Autodesk Inventor part; units mm, degrees
ref_plane "YZ Plane" through (0, 0, 0) normal (1, 0, 0) x (0, 1, 0)
ref_plane "XZ Plane" through (0, 0, 0) normal (0, 1, 0) x (-1, 0, 0)
ref_plane "XY Plane" through (0, 0, 0) normal (0, 0, 1) x (1, 0, 0)
sketch "Sketch1" plane through (0, 0, 0) normal (0, 1, 0) x (-1, 0, 0)
  circle A0 centre (0, 0) radius 3.175
  dimension "d0" = 6.35
extrude "Extrusion1" add sketch "Sketch1" along normal blind 50.8
sketch "Sketch2" plane through (0, 50.8, 0) normal (0, 1, 0) x (1, 0, 0)
  point P0 (0, 0)
  point P1 (0, 0)
hole "Hole1" at (0, 50.8, 0) direction (0, -1, 0) diameter 2.5324 depth 9.525 tip angle 118
thread "Thread1"
sketch "Sketch3" plane through (0, 0, 0) normal (0, -1, 0) x (1, 0, 0)
  point P0 (0, 0)
  point P1 (0, 0)
hole "Hole2" at (0, 0, 0) direction (0, 1, 0) diameter 2.5324 depth 9.525 tip angle 118
thread "Thread2"
properties part number "2inStandoff"
CAD build for the part. Positions are in the model's coordinates, mm. A direction names the side the tool comes from. Coordinates: 2 decimals unless noted, no trailing zeros. Order: outer loops, then holes, each group sorted by start corner. A loop starts at its lowest first (then second) coordinate and runs counter-clockwise, first axis right, second up. Notation, with made-up numbers: (18, 37) - (66, 37) arc R16 cw to (66, 42) - close; hole circle Ø2 at (-7.5, 20). An arc over 180 degrees is marked (long way). Answer in a Markdown table with one row per item.
1. Flat gauge pins, fed straight in: P1, Ø1.5, axis at x = -2, y = 27, coming from the +Z side; P2, Ø2, axis at y = 36.5, z = -2, coming from the +X side. Where does each tip first touch, or does it go through?
Answer:
| item | result |
|---|---|
| P1 | z = 2.92 |
| P2 | x = 3.01 |
2. Slice it at C-C, the plane y = 32. List the corners of the cut face in (x, z) (3 decimals).
Answer:
| item | result |
|---|---|
| outline | circle Ø6.35 at (0, 0) |
3. 3-axis set-ups, long thin cutter, end or side, ignore diameter. For faces 4 (the face through (1.236, 4.829, 0.274)), 5 (the face through (1.236, 45.971, -0.274)), 6 (the face through (-1.4, 50.8, -0.7)): which of +Z, -Z, +X, -X, +Y, -Y reach the whole face in a straight line?
Answer:
| item | result |
|---|---|
| face 4 | -Y |
| face 5 | +Y |
| face 6 | +Z, -Z, +X, -X, +Y |
4. Pull direction X, two halves, no side cores. Call faces 1 (the face through (-1.4, 0, -0.7)), 2 (the face through (-0.215, 10.154, 0.048)), 3 (the face through (0.69, 25.04, 3.1)): +X half, -X half, draft (parallel to the pull), parting line (faces both ways), or undercut.
Answer:
| item | result |
|---|---|
| face 1 | draft |
| face 2 | undercut |
| face 3 | parting line |
5. Drill centre lines: L1, parallel to Z at x = 0, y = 4 (3 decimals); L2, parallel to X at y = 44.5, z = 0.5; L3, parallel to Z at x = -1, y = 6.5. Where is each one in solid material? Low to high. Write a range as from..to.
Answer:
| item | result |
|---|---|
| L1 | -3.175..-1.266, 1.266..3.175 |
| L2 | -3.14..-1.16, 1.16..3.14 |
| L3 | -3.01..-0.78, 0.78..3.01 |
6. Slice it at B-B, the plane z = 2.75. List the corners of the cut face in (x, y), then the cut area to 3 significant figures.
Answer:
| item | result |
|---|---|
| outline | (-1.59, 0) - (1.59, 0) - (1.59, 50.8) - (-1.59, 50.8) - close |
| area | 161 mm² |
7. Slice it at D-D, the plane x = 2. List the corners of the cut face in (y, z).
Answer:
| item | result |
|---|---|
| outline | (0, -2.47) - (50.8, -2.47) - (50.8, 2.47) - (0, 2.47) - close |
8. Slice it at A-A, the plane y = 8. List the corners of the cut face in (x, z) (3 decimals), then the cut area to 3 significant figures.
Answer:
| item | result |
|---|---|
| outline | circle Ø6.35 at (0, 0); hole circle Ø2.532 at (0, 0) |
| area | 26.6 mm² |
